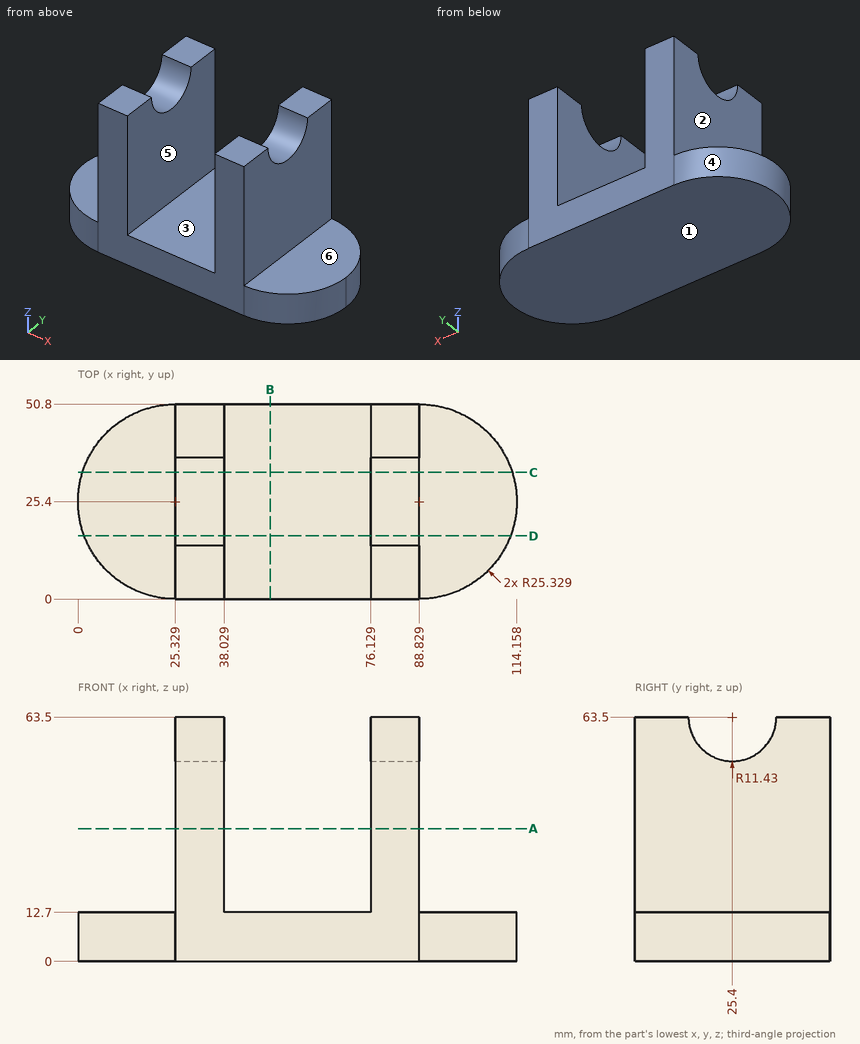
The figure shows three views and two pictorial views of one solid part (mm, origin at its lowest corner). Answer the questions. A direction names the side the tool comes from. Coordinates: 2 decimals unless noted, no trailing zeros. Order: outer loops, then holes, each group sorted by start corner. A loop starts at its lowest first (then second) coordinate and runs counter-clockwise, first axis right, second up. Notation, with made-up numbers: (54.25, 1.25) - (107.25, 1.25) arc R30 cw to (107.25, 29.25) - close; hole circle Ø6 at (17.5, 48). An arc over 180 degrees is marked (long way). Answer as a JSON object with one key per item and string values.
1. Each of these flat-tipped pins is pushed along its axis until it touches: P1, Ø15, axis at y = 25.5, z = 32, coming from the +X side; P2, Ø1.5, axis at y = 24, z = 15.5, coming from the -X side; P3, Ø12.5, axis at x = 96.5, y = 15.5, coming from the +Z side. Where does it stop, or does it pass through?
Output values:
{"P1": "stops at x = 88.83", "P2": "stops at x = 25.33", "P3": "stops at z = 12.7"}
2. Find section D-D on y = 16.5. Determine the outline of the cut face in (x, z) (1 decimal), plus the area to 3 significant figures.
Output values:
{"outline": "(1.6, 0) - (112.5, 0) - (112.5, 12.7) - (88.8, 12.7) - (88.8, 56.3) - (76.1, 56.3) - (76.1, 12.7) - (38, 12.7) - (38, 56.3) - (25.3, 56.3) - (25.3, 12.7) - (1.6, 12.7) - close", "area": "2,520 mm²"}
3. Consider line 1 (X direction, y = 42, z = 42); line 2 (Z direction, x = 48, y = 24); line 3 (Z direction, x = 34, y = 15.5). Determine where each line is inside the solid, lowest interval first.
Output values:
{"line 1": "x = 25.33 to 38.03, 76.13 to 88.83", "line 2": "z = 0 to 12.7", "line 3": "z = 0 to 57.79"}
4. The mould has two halves that part along X. Classify the marked faces 4, 5 and 6: +X half, -X half, draft (parallel to the pull), parting line (faces both ways), or undercut.
Output values:
{"face 4": "-X half", "face 5": "undercut", "face 6": "draft"}
5. A tool of negligible diameter and unlimited length cuts with its end or side. For the marked faces 1, 2 and 3, from which of +Z, -Z, +X, -X, +Y, -Y can it reach the whole face along a straight path? Write none if from no direction.
Output values:
{"face 1": "-Z, +X, -X, +Y, -Y", "face 2": "+Z, -X, +Y, -Y", "face 3": "+Z, +Y, -Y"}
6. Find section B-B on x = 50. Determine the outline of the cut face in (y, z).
Output values:
{"outline": "(0, 0) - (50.8, 0) - (50.8, 12.7) - (0, 12.7) - close"}
7. Find section C-C on y = 33. Determine the outline of the cut face in (x, z), plus the area to 3 significant figures.
Output values:
{"outline": "(1.17, 0) - (112.99, 0) - (112.99, 12.7) - (88.83, 12.7) - (88.83, 54.96) - (76.13, 54.96) - (76.13, 12.7) - (38.03, 12.7) - (38.03, 54.96) - (25.33, 54.96) - (25.33, 12.7) - (1.17, 12.7) - close", "area": "2,490 mm²"}
8. Find section A-A on z = 34.5. Determine the outline of the cut face in (x, y), plus the area to 3 significant figures.
Output values:
{"outline": "(25.33, 0) - (38.03, 0) - (38.03, 50.8) - (25.33, 50.8) - close; (76.13, 0) - (88.83, 0) - (88.83, 50.8) - (76.13, 50.8) - close", "area": "1,290 mm²"}
